The model under review builds one solid part; all positions refer to its coordinate system, in mm. A direction names the side the tool comes from. Coordinates: 2 decimals unless noted, no trailing zeros. Loops run counter-clockwise (first coordinate to the right, second up) from the corner with the lowest first, then second, coordinate; pieces in that order, holes last. Notation, with made-up numbers: (-34.5, -7.5) - (13.5, -7.5) arc R25 cw to (13.5, 9.5) - close; hole circle Ø6 at (-25, 20). An arc over 180 degrees is marked (long way). Use a Markdown table: item, result. Add a question column.
1) Add section B-B, the plane y = 20. Give the boundary of the cut face in (x, z), and give its area (3 significant figures).
2) Clearance check with flat-ended pins moving along their axes: pin 1 (10 mm diameter, centred on y = 16, z = 0, fed in from -X); pin 2 (8 mm diameter, centred on y = 8, z = -44.5, fed in from -X); pin 3 (5 mm diameter, centred on y = 3, z = -51, fed in from -X); pin 4 (2.5 mm diameter, centred on x = 5.15, z = -55, fed in from +Y). State where each tip first meets the part, or that it passes through.
3) The part is to be moulded in two halves that separate along X. For faces 1 (the cylindrical face through (5.177, 2.317, -53.502)), 2 (the flat face through (3, 5, -54)), 3 (the cylindrical face through (-5.775, 9.547, -4.529)), 4 (the cylindrical face through (2.1, 12.32, -44.97)), say which applies: pulls with the +X half, pulls with the -X half, needs draft (parallel to the pull), parting line crosses it, or undercut.
4) To check wall thickness, follow L1, parallel to Z at x = -4, y = 22; L2, parallel to Y at x = -5.25, z = -32; L3, parallel to Z at x = -1.75, y = 10.75. State the ranges of each line that lie inside material, in increasing order. Write a range as [from, to].
5) Add section A-A, the plane y = 11. Give the boundary of the cut face in (x, z), and give its area (3 significant figures).
6) Add section C-C, the plane z = -17.5. Give the boundary of the cut face in (x, y).
7) Add section D-D, the plane y = 17. Give the boundary of the cut face in (x, z), and give its area (3 significant figures).
8) For faces 5 (the cylindrical face through (0.93, 5.713, -1.409)), 6 (the cylindrical face through (-4.09, 17.25, -38.67)), 7 (the cylindrical face through (1.52, 5.71, -50.12)), 8 (the flat face through (2, 5, 3)), list the 3-axis set-ups (+Z, -Z, +X, -X, +Y, -Y) from which the entire face can be reached by the end or side of a thin tool; tool diameter is ignored.
```python
from build123d import *

# Parameters (mm, degrees)
CROQUIS2_R                                           = 1.5000000000000007
SALIENTE_EXTRUIR1_DEPTH                              = 5
SALIENTE_EXTRUIR2_DEPTH                              = 25
AVELLANADO_PARA_TORNILLO_CON_CABEZA_PLAN_D           = 1.8
AVELLANADO_PARA_TORNILLO_CON_CABEZA_PLAN_CSINK_D     = 3.6
AVELLANADO_PARA_TORNILLO_CON_CABEZA_PLAN_CSINK_ANGLE = 90
SALIENTE_EXTRUIR3_DEPTH                              = 25
CORTAR_EXTRUIR3_REACH                                = 53.752
CROQUIS13_W                                          = 29.905861654600464
CROQUIS13_H                                          = 18
CORTAR_EXTRUIR7_DEPTH                                = 57.075529812190766
CORTAR_EXTRUIR7_DEPTH_BACK                           = 16.3
CROQUIS44_W                                          = 16.299999999999983
CROQUIS44_H                                          = 7.0000000000000036
CORTAR_EXTRUIR8_DEPTH                                = 1
REDONDEO1_R                                          = 2.5


with BuildPart() as part:
    # Croquis2 → Saliente-Extruir1 (new body)
    with BuildSketch(Plane(origin=(0, 0, 0), x_dir=(1, 0, 0), z_dir=(0, 1, 0))):
        with BuildLine():
            Line((4.439129900634949, 2.118516979293595), (-4.614530320763677, 2.2280379015268346))
            ThreePointArc((-4.614530320763688, 2.2280379015268323), (-1.7200044543519404, -2.2420294069801585), (1.789858261170167, -6.247106865918674))
            ThreePointArc((1.7898582611701688, -6.247106865918663), (7.12266646558417, -6.2115073036702295), (7.087066903335739, -0.8786990992562278))
            ThreePointArc((7.087066903335739, -0.8786990992562309), (5.711774187433154, 0.574565767125705), (4.439129900634946, 2.118516979293595))
        make_face()
        with Locations(Location((4.438462582252952, -3.5629029825874476, 0), (0, 0, 270))):
            Circle(CROQUIS2_R, mode=Mode.SUBTRACT)
    extrude(amount=SALIENTE_EXTRUIR1_DEPTH)

    # Croquis2_3 → Saliente-Extruir2 (add)
    with BuildSketch(Plane(origin=(0, 0, 0), x_dir=(1, 0, 0), z_dir=(0, 1, 0))):
        with BuildLine():
            ThreePointArc((-8.348947802254838, 12.273944296748217), (-6.849717496148568, 7.114200545347133), (-4.614530320763688, 2.2280379015268323))
            Line((-4.614530320763677, 2.2280379015268346), (4.439129900634949, 2.118516979293595))
            ThreePointArc((4.439129900634946, 2.118516979293595), (1.4480092130333588, 6.906303569503548), (-0.566904192020619, 12.179805951348676))
            Line((-0.5669041920206155, 12.179805951348678), (-8.348947802254829, 12.273944296748219))
        make_face()
    extrude(amount=SALIENTE_EXTRUIR2_DEPTH)

    # Avellanado para tornillo con cabeza plan (through all)
    with Locations(Plane(origin=(0, 5, 0), x_dir=(1, 0, 0), z_dir=(0, 1, 0))):
        with Locations((4.438462582, -3.562902983)):
            CounterSinkHole(AVELLANADO_PARA_TORNILLO_CON_CABEZA_PLAN_D / 2, AVELLANADO_PARA_TORNILLO_CON_CABEZA_PLAN_CSINK_D / 2, counter_sink_angle=AVELLANADO_PARA_TORNILLO_CON_CABEZA_PLAN_CSINK_ANGLE)

    # Croquis8 → Saliente-Extruir3 (add)
    with BuildSketch(Plane(origin=(0, 0, 0), x_dir=(1, 0, 0), z_dir=(0, 1, 0))):
        Polygon((-8.348947802254834, 42.17980595134868), (-0.5669041920206199, 42.085667605949155), (-0.5669041920206147, 12.179805951348678), (-8.348947802254829, 12.273944296748219), align=None)
    extrude(amount=SALIENTE_EXTRUIR3_DEPTH)

    # Croquis13 → Cortar-Extruir3 (cut, up to next)
    with BuildSketch(Plane.ZY.offset(8.348947802254827), mode=Mode.PRIVATE) as cortar_extruir3_sk1:
        with Locations((-27.22687512404845, 9)):
            Rectangle(CROQUIS13_W, CROQUIS13_H)
    cortar_extruir3_tool1 = extrude(cortar_extruir3_sk1.sketch, amount=-CORTAR_EXTRUIR3_REACH, mode=Mode.PRIVATE) & part.part
    add(cortar_extruir3_tool1.solids().sort_by_distance((-8.348948, 9, -27.226875))[0], mode=Mode.SUBTRACT)

    # Croquis42 → Cortar-Extruir7 (cut, two sides: drawn at the far end of the back side and taken through both)
    with BuildSketch(Plane(origin=(0.5089472836094107, 0, -42.072653173894544), x_dir=(-0.9999268409353232, 0, -0.012095981857829284), z_dir=(0.012095981857829284, 0, -0.9999268409353232)).offset(-CORTAR_EXTRUIR7_DEPTH_BACK)):
        Polygon((1.0759301896763651, 88.39893602181824), (1.0759301896763651, 25), (1.0759301896763651, 18), (8.85854316859686, 18), (72.2574791904151, 18), (161.42014152905733, 108.15386846652605), (90.2385925283186, 178.5528044883443), align=None)
    extrude(amount=CORTAR_EXTRUIR7_DEPTH + CORTAR_EXTRUIR7_DEPTH_BACK, mode=Mode.SUBTRACT)

    # Croquis44 → Cortar-Extruir8 (cut)
    with BuildSketch(Plane(origin=(-1.0758514756300315, 0, -0.01301443205461614), x_dir=(-0.012095981857829285, 0, 0.9999268409353232), z_dir=(-0.9999268409353232, 0, -0.012095981857829285))):
        with Locations((-33.92573139504898, 21.5)):
            Rectangle(CROQUIS44_W, CROQUIS44_H)
    extrude(amount=-CORTAR_EXTRUIR8_DEPTH, mode=Mode.SUBTRACT)

    # Redondeo1
    redondeo1_edges = [part.edges().sort_by_distance(p)[0] for p in [
        (-4.457925997137721, 0, -12.273944296748217),
        (-4.457925997137721, 18, -12.273944296748217),
        (-0.08770021006436401, 5, -2.1732774404102146),
        (-0.08770021006436401, 25, -2.1732774404102146),
    ]]
    fillet(redondeo1_edges, radius=REDONDEO1_R)

    # Simetr_a1: part across plane


with BuildPart() as part_1:
    add(part.part)
    add(part.part.mirror(Plane(origin=(-8.546112306537452, 25, -25.88099844410291), x_dir=(0.9999268409353231, 0, 0.012095981857829284), z_dir=(-0.012095981857829282, 0, 0.9999268409353232))))


solid = part_1.part
```
From the geometry:
| question | item | result |
|---|---|---|
| 1 | outline | (-8.35, -25.88) - (-8.02, -39.48) arc R36.77 ccw to (-4.04, -49.43) - (5.01, -49.32) arc R29.23 cw to (-0.24, -39.39) - (-0.57, -25.78) - (-0.57, -12.18) arc R29.23 cw to (4.44, -2.12) - (-4.61, -2.23) arc R36.77 ccw to (-8.35, -12.27) - close |
| 1 | area | 378 mm^2 |
| 2 | pin 1 | stops at x = -5.99 |
| 2 | pin 2 | stops at x = -7.76 |
| 2 | pin 3 | stops at x = -4.57 |
| 2 | pin 4 | passes through |
| 3 | face 1 | undercut |
| 3 | face 2 | needs draft |
| 3 | face 3 | pulls with the -X half |
| 3 | face 4 | pulls with the +X half |
| 4 | L1 | z = [-49.43, -2.22] |
| 4 | L2 | y = [18, 25] |
| 4 | L3 | z = [-49.4, -39.33], [-12.27, -2.19] |
| 5 | outline | (-8.35, -12.27) - (-0.57, -12.27) - (-0.57, -12.18) arc R29.23 cw to (4.44, -2.12) - (-4.61, -2.23) arc R36.77 ccw to start; (-8.02, -39.48) arc R36.77 ccw to (-4.04, -49.43) - (5.01, -49.32) arc R29.23 cw to (-0.24, -39.39) - (-0.24, -39.29) - close |
| 5 | area | 167 mm^2 |
| 6 | outline | (-8.35, 18) - (-0.57, 18) - (-0.57, 25) - (-8.35, 25) - close |
| 7 | outline | (-8.35, -12.77) - (-0.57, -12.77) - (-0.57, -12.18) arc R29.23 cw to (4.44, -2.12) - (-4.61, -2.23) arc R36.77 ccw to (-8.35, -12.27) - close; (-8.03, -38.98) - (-8.02, -39.48) arc R36.77 ccw to (-4.04, -49.43) - (5.01, -49.32) arc R29.23 cw to (-0.24, -39.39) - (-0.25, -38.79) - close |
| 7 | area | 174 mm^2 |
| 8 | face 5 | +Z, -X, +Y |
| 8 | face 6 | -X, -Y |
| 8 | face 7 | -Z, +X, +Y |
| 8 | face 8 | +Z, +X, -X, +Y |
